For this review, take the finished solid that the model builds, in its own axes (mm). Face numbers are marked on the shaded views. A direction names the side the tool comes from. Round coordinates to 2 decimals unless told otherwise and drop trailing zeros. Write each loop counter-clockwise with the first axis right and the second up, starting at its lowest first coordinate (ties: lowest second). Pieces come first, ordered by that corner, then holes. Notation, with made-up numbers: M 31.25,20 L 58.25,20 A22 ccw 58.25,46 Z; hole C -17,61.25 d4. An arc over 180 degrees is marked long. Use one line per item in the form item = value. Start each with the question number.
Item 1: For the marked faces 1 and 2, list the 3-axis set-ups (+Z, -Z, +X, -X, +Y, -Y) from which the entire face can be reached by the end or side of a thin tool; tool diameter is ignored.
Item 2: For line 1 (Y direction, x = 10.5, z = 5.1); line 2 (Y direction, x = -11.5, z = 5); line 3 (X direction, y = 11, z = 1.9), list the stretches that pass through material, from the lowest coordinate up. Write a range as [from, to].
Item 3: Add section C-C (z = 2.1). State the section outline as (x, y) points.
Item 4: For P1, Ø1, axis at x = -9, y = 0.5, coming from the -Z side; P2, Ø5.5, axis at x = -2.5, y = 10, coming from the -Z side; P3, Ø8, axis at x = 3, y = 6, coming from the +Z side, all flat-tipped, find the tip position at first contact; note any pin that passes through.
from build123d import *

# Parameters (mm, degrees)
EXTRUDE_2_DEPTH = 0.4


with BuildPart() as part:
    # Sketch 1 → Revolve 2 (revolve)
    with BuildSketch(Plane(origin=(0, 0, 0), x_dir=(1, 0, 0), z_dir=(0, 1, 0)), mode=Mode.PRIVATE) as revolve_2_sk:
        with BuildLine():
            Line((0, 0), (7.5, 0))
            ThreePointArc((7.5, 0), (7.853553391, -0.146446609), (8, -0.5))
            Line((8, -0.5), (8, -1.5))
            Line((8, -1.5), (12.25, -1.5))
            ThreePointArc((12.25, -1.5), (12.957106781, -1.792893219), (13.25, -2.5))
            Line((13.25, -2.5), (13.25, -3))
            Line((13.25, -3), (13.5, -3))
            ThreePointArc((13.5, -3), (13.853553391, -3.146446609), (14, -3.5))
            Line((14, -3.5), (14, -4.4))
            Line((14, -4.4), (13.5, -4.4))
            Line((13.5, -4.4), (13.5, -5.4))
            Line((13.5, -5.4), (12.7, -5.4))
            Line((12.7, -5.4), (12.7, -4.1))
            Line((12.7, -4.1), (12, -4.1))
            ThreePointArc((12, -4.1), (9.5, -5), (7, -4.1))
            ThreePointArc((7, -4.1), (3.528809998, -4.77407776), (0, -5))
            Line((0, -5), (0, 0))
        make_face()
    revolve(revolve_2_sk.sketch.rotate(Axis((0, 0, 0), (0, 0, 1)), 180), axis=Axis((0, 0, 0), (0, 0, 1)))

    # Sketch 2 → Extrude 2 (add)
    with BuildSketch(Plane(origin=(0, 0, 1.5), x_dir=(-1, 0, 0), z_dir=(0, 0, -1))):
        with BuildLine():
            Line((-5.564516129, 6.589900246), (-7.5, 8.882039462))
            ThreePointArc((-7.5, 8.882039462), (0, 11.625), (7.5, 8.882039462))
            Line((7.5, 8.882039462), (5.564516129, 6.589900246))
            ThreePointArc((5.564516129, 6.589900246), (0, 8.625), (-5.564516129, 6.589900246))
        make_face()
    extrude(amount=EXTRUDE_2_DEPTH)


solid = part.part
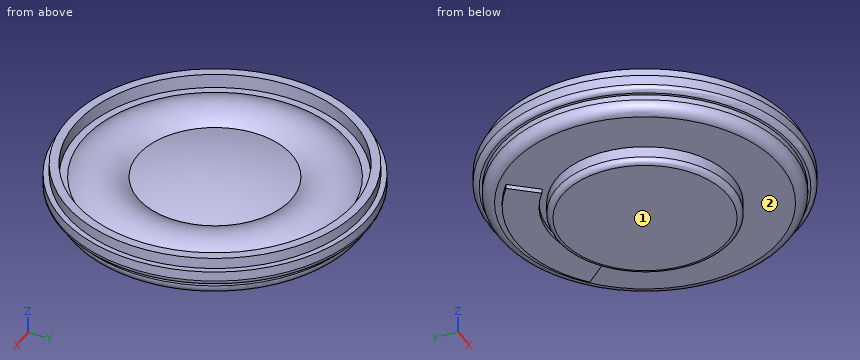
Calculated:
q1.face_1 = -Z, +X, -X, +Y, -Y
q1.face_2 = -Z
q2.line_1 = [-8.49, -7.14], [7.14, 8.49]
q2.line_2 = [-7.07, -5.39], [5.39, 7.07]
q2.line_3 = [-7.02, 7.02]
q3.outline = C 0,0 d26.33
q4.P1 = 1.5
q4.P2 = 0
q4.P3 = 5
